Autodesk Inventor part; units mm, degrees
ref_plane "YZ Plane" through (0, 0, 0) normal (1, 0, 0) x (0, 1, 0)
ref_plane "XZ Plane" through (0, 0, 0) normal (0, 1, 0) x (-1, 0, 0)
ref_plane "XY Plane" through (0, 0, 0) normal (0, 0, 1) x (1, 0, 0)
ref_plane "Plano de trabajo1" through (0, 0, 0) normal (0, 0, 1) x (1, 0, 0)
sketch "Boceto1" plane through (0, 0, 0) normal (0, 0, 1) x (1, 0, 0)
  circle A0 centre (10.9923, 0) radius 10.9823
  circle A1 centre (10.9923, 7.35) radius 1.2028
  circle A2 centre (3.6423, 0) radius 1.2028
  circle A3 centre (18.3423, 0) radius 1.2028
  circle A4 centre (18.7153, -9.5116) radius 1.05
  circle A5 centre (10.9923, -7.35) radius 1.2028
  line L0 (10.9923, 0) -> (160.9923, 0)
  line L1 (10.9923, 10.9823) -> (160.9923, 10.9823)
  line L2 (10.9923, -10.9823) -> (160.9923, -10.9823)
  line L3 (160.9923, -10.9823) -> (160.9923, 10.9823)
  point P0 (0, 0)
  dimension "d0" = 150
extrude "Extrusión1" add sketch "Boceto1" along normal blind 3
sketch "Boceto2" plane through (0, 0, 3) normal (0, 0, 1) x (1, 0, 0)
  arc A0 (151.1597, 5.5871) -> (154.1073, 8.4343) centre (150.0864, 9.6477) ccw
  circle A1 centre (150.0864, -8.5523) radius 0.85
  circle A2 centre (150.0864, 9.6477) radius 0.85
  line L0 (160.9923, 10.9823) -> (10.9923, 10.9823)
  line L1 (10.9923, -10.9823) -> (160.9923, -10.9823)
  line L2 (160.9923, -10.9823) -> (160.9923, 10.9823)
  line L3 (160.9923, 10.9823) -> (10.9923, 10.9823)
  arc A3 (10.9923, 10.9823) -> (10.9923, -10.9823) centre (10.9923, 0) ccw
  circle A4 centre (18.7153, -9.5116) radius 1.05
  circle A5 centre (10.9923, 7.35) radius 1.2028
  circle A6 centre (3.6423, 0) radius 1.2028
  circle A7 centre (10.9923, -7.35) radius 1.2028
  circle A8 centre (18.3423, 0) radius 1.2028
  line L4 (150.0864, 10.9823) -> (150.0864, -0.0002)
  line L5 (150.0864, -0.0002) -> (150.0864, -9.1002)
  line L6 (150.0864, -0.0002) -> (150.0864, 9.0998)
  circle A9 centre (150.0864, 9.0998) radius 0.85
  circle A10 centre (150.0864, -9.1002) radius 0.85
  circle A11 centre (150.0864, 9.0998) radius 1.8825
  circle A12 centre (150.0864, -9.1002) radius 1.8821
  point P0 (0, 0)
  point P1 (150.0864, 7.2173)
  point P2 (150.0864, -7.218)
  point P3 (150.0864, -10.9823)
  dimension "d3" = 10.9825
  dimension "d4" = 9.1
  dimension "d5" = 9.1
  dimension "d6" = 1.7
  dimension "d7" = 1.7
extrude "Extrusión2" cut sketch "Boceto2" against normal blind 3 contours L5 L4 A11 L0 L2 L1 A12 | A10 A1 | A1 A10 | A9 A2 L4 | L4 A2 A9 | L4 A9 A2 | A2 A9 L4 picked at (149.9501, 8.6317) picked at (150.2191, 8.6309) picked at (150.5614, 9.2824) picked at (149.6114, 9.2824)
sketch "Boceto3" plane through (0, 0, 3) normal (0, 0, 1) x (1, 0, 0)
  point P0 (0, 0)
sketch "Boceto4" plane through (0, 0, 3) normal (0, 0, 1) x (1, 0, 0)
  circle A0 centre (18.7153, -9.5116) radius 1.05
  point P0 (0, 0)
extrude "Extrusión3" add sketch "Boceto4" against normal blind 3
properties part number "tibiaMot"
Input: part model. Units: mm. Frame: model coordinates. A direction names the side the tool comes from. Coordinates: 2 decimals unless noted, no trailing zeros. Loops run counter-clockwise (first coordinate to the right, second up) from the corner with the lowest first, then second, coordinate; pieces in that order, holes last. Notation, with made-up numbers: (39, 20.5) -> (81, 20.5) arc R8 ccw to (81, 29.5) -> close; hole circle Ø7 at (18, 28). An arc over 180 degrees is marked (long way). One line per item, written item: value.
(1) Ray query, line 1 along X through (y, z) = (9.25, 1.05); line 2 along X through (y, z) = (-1, 1.15); line 3 along X through (y, z) = (5, 1.55). Return the intervals inside material, ascending.
Answer below:
line 1: x = 5.07 to 149.25, 150.92 to 151.96
line 2: x = 0.06 to 2.97, 4.31 to 17.67, 19.01 to 150.09
line 3: x = 1.21 to 150.09
(2) Draft query along X for faces 1 (the face through (0.013, -0.241, 1.479)), 2 (the face through (151.97, -9.14, 1.52)), 3 (the face through (19.49, -0.36, 1.48)), 4 (the face through (2.44, -0.05, 1.48)). Return one class per face: pulls with the +X half, pulls with the -X half, needs draft (parallel to the pull), parting line crosses it, or undercut.
Answer below:
face 1: pulls with the -X half
face 2: pulls with the +X half
face 3: undercut
face 4: undercut
(3) Set-up query: faces 5 (the face through (80, 10.982, 1)), 6 (the face through (150.086, 0, 2)). Return all of +Z, -Z, +X, -X, +Y, -Y with unobstructed straight access to the full face (end or side cutting, diameter ignored); none if empty.
Answer below:
face 5: +Z, -Z, +X, -X, +Y
face 6: +Z, -Z, +X
(4) Pin query (flat end, axial travel): pin 1 Ø0.9 at (y, z) = (0.5, 1) entering from +X. Return the tip coordinate at first contact, or that it passes through.
Answer below:
pin 1: stops at x = 150.09
(5) Cut plane A-A (z = 2.25). Give the number of separate pieces and of enclosed holes in the cut face, then the cut area to 3 significant figures.
Answer below:
separate pieces: 1
enclosed holes: 6
area: 3,230 mm2
(6) Cut plane B-B (y = -3.25). Output: boundary loops of the cut face in (x, z).
Answer below:
outline: (0.5, 0) -> (150.09, 0) -> (150.09, 3) -> (0.5, 3) -> close
